from build123d import *

# Parameters (mm, degrees)
SKETCH1_W                         = 32
SKETCH1_H                         = 29
BOSS_EXTRUDE1_DEPTH               = 35
FILLET1_R                         = 2
SLOT_FOR_COIL_DEPTH               = 1
SLOT_FOR_COIL_DEPTH_BACK          = 30
BOSS_EXTRUDE2_DEPTH               = 7
BOSS_EXTRUDE3_DEPTH               = 1.75
SKETCH5_W                         = 2
SKETCH5_H                         = 7
SLOT_TO_FEED_IN_WIRE_DEPTH        = 33
SLOT_FO_PCB_DEPTH                 = 22
SKETCH7_W                         = 2
SKETCH7_H                         = 33
BOSS_EXTRUDE4_DEPTH               = 0.25
FILLET2_R                         = 6
ROD_MOUNT_SLOT_REACH              = 34
SKETCH14_W                        = 2.5
SKETCH14_H                        = 20
SIDE_CAVITY_FOR_MOUNT_PLATE_DEPTH = 22
SKETCH16_W                        = 2
SKETCH16_H                        = 2
SIDE_STOPS_FOR_MOUNT_PLATE_DEPTH  = 22
BOSS_EXTRUDE6_DEPTH               = 22
SKETCH21_W                        = 12
SKETCH21_H                        = 2
BOSS_EXTRUDE7_DEPTH               = 4
SKETCH23_W                        = 8
SKETCH23_H                        = 1.75
CUT_EXTRUDE7_DEPTH                = 2
FILLET3_R                         = 1
CUT_EXTRUDE8_REACH                = 34
SKETCH26_R                        = 5.5


with BuildPart() as part:
    # Sketch1 → Boss-Extrude1 (new body)
    with BuildSketch(Plane.XY):
        Rectangle(SKETCH1_W, SKETCH1_H)
    extrude(amount=BOSS_EXTRUDE1_DEPTH)

    # Fillet1
    fillet1_edges = [part.edges().sort_by_distance(p)[0] for p in [
        (16, -14.5, 17.5),
        (-16, -14.5, 17.5),
        (-16, 14.5, 17.5),
        (16, 14.5, 17.5),
    ]]
    fillet(fillet1_edges, radius=FILLET1_R)

    # Sketch2 → Slot for Coil (cut, two sides)
    with BuildSketch(Plane.XZ.offset(14.5)) as slot_for_coil_sk:
        Polygon((-9.125, 0), (-9.125, 1.75), (-11.125, 1.75), (-11.125, 5), (11.125, 5), (11.125, 1.75), (9.125, 1.75), (9.125, 0), align=None)
    extrude(amount=SLOT_FOR_COIL_DEPTH, mode=Mode.SUBTRACT)
    extrude(slot_for_coil_sk.sketch, amount=-SLOT_FOR_COIL_DEPTH_BACK, mode=Mode.SUBTRACT)

    # Sketch3 → Boss-Extrude2 (add)
    with BuildSketch(Plane.XZ.offset(14.5)):
        Polygon((-9.125, 0), (-9.125, 1.75), (-11.125, 1.75), (-11.125, 5), (11.125, 5), (11.125, 1.75), (9.125, 1.75), (9.125, 0), align=None)
    extrude(amount=-BOSS_EXTRUDE2_DEPTH)

    # Sketch4 → Boss-Extrude3 (add)
    with BuildSketch(Plane(origin=(0, 0, 1.75), x_dir=(-1, 0, 0), z_dir=(0, 0, -1))):
        with BuildLine():
            Line((-9.125, 7.5), (-9.125, 6.5))
            ThreePointArc((-9.125, 6.5), (-8.875, 7), (-9.125, 7.5))
        make_face()
    boss_extrude3 = extrude(amount=BOSS_EXTRUDE3_DEPTH)

    # Mirror1: Boss-Extrude3 across plane
    add(boss_extrude3.mirror(Plane(origin=(0, 0, 0), x_dir=(0, 0, 1), z_dir=(1, 0, 0))))

    # Sketch5 → slot to feed in wire (cut)
    with BuildSketch(Plane(origin=(0, 0, 0), x_dir=(-1, 0, 0), z_dir=(0, 0, -1))):
        with Locations((0, -11)):
            Rectangle(SKETCH5_W, SKETCH5_H)
    extrude(amount=-SLOT_TO_FEED_IN_WIRE_DEPTH, mode=Mode.SUBTRACT)

    # Sketch6 → slot fo PCB (cut)
    with BuildSketch(Plane(origin=(0, 14.5, 0), x_dir=(1, 0, 0), z_dir=(0, 1, 0))):
        Polygon((11.5, -7.5), (-11.5, -7.5), (-11.5, -29.5), (-12.5, -29.5), (-12.5, -33), (12.5, -33), (12.5, -29.5), (11.5, -29.5), align=None)
    extrude(amount=-SLOT_FO_PCB_DEPTH, mode=Mode.SUBTRACT)

    # Sketch7 → Boss-Extrude4 (add)
    with BuildSketch(Plane.XZ.offset(14.5)):
        with Locations((0, 16.5)):
            Rectangle(SKETCH7_W, SKETCH7_H)
    extrude(amount=-BOSS_EXTRUDE4_DEPTH)

    # Fillet2
    fillet2_edges = [part.edges().sort_by_distance(p)[0] for p in [
        (0, -14.25, 33),
    ]]
    fillet(fillet2_edges, radius=FILLET2_R)

    # Sketch11 → Rod Mount Slot (cut, up to next)
    with BuildSketch(Plane(origin=(16, 0, 44), x_dir=(0, 0, -1), z_dir=(1, 0, 0)), mode=Mode.PRIVATE) as rod_mount_slot_sk1:
        with BuildLine():
            Line((32.5, 25), (32.5, 0))
            ThreePointArc((32.5, 0), (26.5, -6), (20.5, 0))
            Line((20.5, 0), (20.5, 25))
            ThreePointArc((20.5, 25), (26.5, 31), (32.5, 25))
        make_face()
    rod_mount_slot_tool1 = extrude(rod_mount_slot_sk1.sketch, amount=-ROD_MOUNT_SLOT_REACH, mode=Mode.PRIVATE) & part.part
    add(rod_mount_slot_tool1.solids().sort_by_distance((16, 12.5, 17.5))[0], mode=Mode.SUBTRACT)

    # Sketch14 → Side cavity for mount plate (cut)
    with BuildSketch(Plane(origin=(0, 14.5, 0), x_dir=(1, 0, 0), z_dir=(0, 1, 0))):
        with Locations((12.75, -17.5)):
            Rectangle(SKETCH14_W, SKETCH14_H)
    extrude(amount=-SIDE_CAVITY_FOR_MOUNT_PLATE_DEPTH, mode=Mode.SUBTRACT)

    # Sketch16 → Side stops for mount plate (add)
    with BuildSketch(Plane(origin=(0, 14.5, 0), x_dir=(1, 0, 0), z_dir=(0, 1, 0))):
        with Locations((11, -8.5)):
            Rectangle(SKETCH16_W, SKETCH16_H)
        with Locations((11, -26.5)):
            Rectangle(SKETCH16_W, SKETCH16_H)
    extrude(amount=-SIDE_STOPS_FOR_MOUNT_PLATE_DEPTH)

    # Sketch20 → Boss-Extrude6 (add)
    with BuildSketch(Plane(origin=(0, 14.5, 0), x_dir=(1, 0, 0), z_dir=(0, 1, 0))):
        Polygon((11.5, -29.5), (10, -27.5), (11.5, -27.5), align=None)
        Polygon((10, -9.5), (8.5, -7.5), (10, -7.5), align=None)
    extrude(amount=-BOSS_EXTRUDE6_DEPTH)

    # Sketch21 → Boss-Extrude7 (add)
    with BuildSketch(Plane(origin=(0, 14.5, 0), x_dir=(-1, 0, 0), z_dir=(0, 1, 0))):
        with Locations((0, 34)):
            Rectangle(SKETCH21_W, SKETCH21_H)
    boss_extrude7 = extrude(amount=BOSS_EXTRUDE7_DEPTH)

    # Sketch23 → Cut-Extrude7 (cut)
    with BuildSketch(Plane.XY.offset(35)):
        with Locations((0, 15.875)):
            Rectangle(SKETCH23_W, SKETCH23_H)
    cut_extrude7 = extrude(amount=-CUT_EXTRUDE7_DEPTH, mode=Mode.SUBTRACT)

    # Mirror3: Boss-Extrude7, Cut-Extrude7 across plane
    add(boss_extrude7.mirror(Plane.ZX))
    add(cut_extrude7.mirror(Plane.ZX), mode=Mode.SUBTRACT)

    # Fillet3
    fillet3_edges = [part.edges().sort_by_distance(p)[0] for p in [
        (6, 14.5, 34),
        (-6, 14.5, 34),
        (6, 18.5, 34),
        (-6, 18.5, 34),
        (6, -18.5, 34),
        (-6, -18.5, 34),
        (6, -14.5, 34),
        (-6, -14.5, 34),
    ]]
    fillet(fillet3_edges, radius=FILLET3_R)

    # Sketch26 → Cut-Extrude8 (cut, up to next)
    with BuildSketch(Plane(origin=(-16, 0, 0), x_dir=(0, 0, -1), z_dir=(1, 0, 0)), mode=Mode.PRIVATE) as cut_extrude8_sk1:
        with Locations((-23.015, -2.89)):
            Circle(SKETCH26_R)
    cut_extrude8_tool1 = extrude(cut_extrude8_sk1.sketch, amount=CUT_EXTRUDE8_REACH, mode=Mode.PRIVATE) & part.part
    add(cut_extrude8_tool1.solids().sort_by_distance((-16, -2.89, 23.015))[0], mode=Mode.SUBTRACT)


solid = part.part
Geometry: final body of the model. Coordinates: model frame, mm. A direction names the side the tool comes from. Give positions to 0.01 mm unless a question says otherwise; leave off trailing zeros. Write each loop counter-clockwise with the first axis right and the second up, starting at its lowest first coordinate (ties: lowest second). Pieces come first, ordered by that corner, then holes. Notation, with made-up numbers: M 62.25,6.5 L 74.25,6.5 A10 cw 74.25,24.5 Z; hole C 71,7.5 d7. An arc over 180 degrees is marked long. Answer in a Markdown table with one row per item. Add a question column.
(1) Ray query, line 1 (X direction, y = 7, z = 27); line 2 (Z direction, x = -10.5, y = -2.89); line 3 (X direction, y = -8, z = 27). Return the intervals inside material, ascending.
(2) Section B-B on y = -16. Return loops of the section in (x, z).
(3) Reachability of faces 4 (the flat face through (0, -16.75, 34)), 5 (the flat face through (-12.5, 4, 31)), 6 (the flat face through (6, 16, 34)) from +Z, -Z, +X, -X, +Y, -Y: full face, straight path, thin tool, end or side. Return the list, or none.
(4) Mould query, pull axis Y, two halves, no side actions, for faces 1 (the flat face through (-4, -10, 0)), 2 (the flat face through (0, -18.5, 34)), 3 (the flat face through (-4, 16, 34)). Classes: +Y half, -Y half, draft (parallel to the pull), parting line (faces both ways), or undercut.
(5) Section A-A on x = -2. Return loops of the section in (y, z) (3 decimals).
(6) Section D-D on z = 31. Return loops of the section in (x, y), and give its area (3 significant figures).
(7) First-contact query: pin 1 (2 mm diameter, centred on x = -1.5, z = 23.5, fed in from +Y); pin 2 (6.5 mm diameter, centred on y = 6, z = 17, fed in from +X); pin 3 (1 mm diameter, centred on x = -2, z = 31, fed in from +Y). Flat tips, straight axial feed; report the tip coordinate or a pass-through.
Result set:
| question | item | result |
|---|---|---|
| 1 | line 1 | x = -16 to -11.5, 10 to 12, 14 to 16 |
| 1 | line 2 | z = 0 to 1.75, 5 to 7.5, 33 to 35 |
| 1 | line 3 | x = -16 to -1, 1 to 16 |
| 2 | outline | M -6,33 L -4,33 L -4,35 L -6,35 Z; M 4,33 L 6,33 L 6,35 L 4,35 Z |
| 3 | face 4 | +Z, -Z |
| 3 | face 5 | +Y |
| 3 | face 6 | +Z, -Z, +X, +Y |
| 4 | face 1 | draft |
| 4 | face 2 | -Y half |
| 4 | face 3 | undercut |
| 5 | outline | M -18.5,33 L -16.75,33 L -16.75,35 L -18.5,35 Z; M -15,33 L -14.5,33 L -14.5,0 L -7.5,0 L -7.5,5 L 14.5,5 L 14.5,7.5 L -7.5,7.5 L -7.5,20.015 A5.5 cw -7.5,26.015 L -7.5,33 L 15,33 L 15,35 L -15,35 Z; M 16.75,33 L 18.5,33 L 18.5,35 L 16.75,35 Z |
| 6 | outline | M -16,-12.5 A2 ccw -14,-14.5 L 14,-14.5 A2 ccw 16,-12.5 L 16,12.5 A2 ccw 14,14.5 L 12.5,14.5 L 12.5,-7.5 L 1,-7.5 L 1,-12.72 L -1,-12.72 L -1,-7.5 L -12.5,-7.5 L -12.5,14.5 L -14,14.5 A2 ccw -16,12.5 Z |
| 6 | area | 364 mm^2 |
| 7 | pin 1 | stops at y = -8.19 |
| 7 | pin 2 | stops at x = -11.5 |
| 7 | pin 3 | stops at y = -7.5 |
